Work out the finished part from the listing and answer in its coordinate system (mm). A direction names the side the tool comes from. Coordinates: 2 decimals unless noted, no trailing zeros. Loops run counter-clockwise (first coordinate to the right, second up) from the corner with the lowest first, then second, coordinate; pieces in that order, holes last. Notation, with made-up numbers: (-33.75, 33.5) -> (22.25, 33.5) arc R20 cw to (22.25, 54.5) -> close; hole circle Ø5 at (9, 21.25). An arc over 180 degrees is marked (long way). Use a Markdown table: item, result. Add a question column.
```python
from build123d import *

# Parameters (mm, degrees)
BOSS_EXTRUDE1_DEPTH = 10
SKETCH3_R           = 0.8
CUT_EXTRUDE1_DEPTH  = 10
SHELL3_START        = 0.5
SHELL3_DEPTH        = 9


# Read off the part's stored shape, not the designer's step: Shell3
with BuildPart() as part:
    # Sketch1 → Boss-Extrude1 (new body)
    with BuildSketch(Plane.XY):
        Polygon((0, 0), (17.18164136, 13.403124393), (36.182713788, 0), (31.388050652, 0), (17.18164136, 10.021027584), (3.469055949, -0.675941592), align=None)
    extrude(amount=BOSS_EXTRUDE1_DEPTH)

    # Sketch3 → Cut-Extrude1 (cut)
    with BuildSketch(Plane.XY.offset(10)):
        with Locations((3.03145353, 0.822261973)):
            Circle(SKETCH3_R)
    extrude(amount=-CUT_EXTRUDE1_DEPTH, mode=Mode.SUBTRACT)

    # Shell3 outline → Shell3 (cut)
    with BuildSketch(Plane.XY.offset(SHELL3_START)):
        with BuildLine():
            ThreePointArc((2.871909903, 1.606191709), (3.523511931, 0.19148584), (2.309922075, 1.167793967))
            Line((2.309922075, 1.167793967), (0.650444145, -0.126738299))
            Line((0.650444145, -0.126738299), (2.818611804, -0.549203293))
            Line((2.818611804, -0.549203293), (17.16665434, 10.643475851))
            Line((17.16665434, 10.643475851), (31.546653635, 0.5))
            Line((31.546653635, 0.5), (34.606450873, 0.5))
            Line((34.606450873, 0.5), (17.196628379, 12.780676126))
            Line((17.196628379, 12.780676126), (2.871909903, 1.606191709))
        make_face()
    extrude(amount=SHELL3_DEPTH, mode=Mode.SUBTRACT)


solid = part.part
```
Item 1: Find the intervals of material crossed by probe 1 along X at (y, z) = (5.75, 6.75); probe 2 along X at (y, z) = (3.5, 9.25); probe 3 along Z at (x, y) = (23.5, 8), in increasing order.
Item 2: Given pin 1 (1.5 mm diameter, centred on x = 25, y = 9, fed in from -Z); pin 2 (1 mm diameter, centred on x = 13, z = 6, fed in from -Y); pin 3 (5.5 mm diameter, centred on x = 35, z = 6.5, fed in from -Y); pin 4 (5 mm diameter, centred on y = 8, z = 1.5, fed in from -X), each flat-ended and moving along its own axis, determine where each tip first touches the part or whether it passes through.
Item 3: Section A-A (y = 4.25) is taken. Determine the outline of the cut face in (x, z).
Item 4: For faces 1 (the face through (1.49, 0.53, 4.94)), 2 (the face through (24.384, 4.94, 4.93)), 3 (the face through (21, 8, 0)), 4 (the face through (10.13, 7.27, 4.94)), 5 (the face through (26.549, 6.795, 4.93)), determine the directions among +Z, -Z, +X, -X, +Y, -Y from which every point of the face is accessible in a straight line to the end or side of a thin tool.
Item 5: Section B-B (x = 22) is taken. Determine the outline of the cut face in (y, z), then the cut area to 3 significant figures.
Item 6: Section D-D (x = 34) is taken. Determine the outline of the cut face in (y, z), then the cut area to 3 significant figures.
Item 7: For a pull along Y with two mould halves and no side action, classify faces 6 (the face through (20, 9, 0.5)), 7 (the face through (2.56, 1.47, 5.02)), 8 (the face through (21, 8, 10)), 9 (the face through (34, 0, 5)) as +Y half, -Y half, draft (parallel to the pull), parting line (faces both ways), or undercut.
Item 8: Section C-C (z = 4.75) is taken. Determine the outline of the cut face in (x, y).
Output:
| question | item | result |
|---|---|---|
| 1 | probe 1 | x = 7.37 to 8.18, 10.89 to 11.71, 23.24 to 24.1, 27.16 to 28.03 |
| 1 | probe 2 | x = 4.49 to 5.3, 8.01 to 8.82, 26.43 to 27.29, 30.35 to 31.22 |
| 1 | probe 3 | z = 0 to 0.5, 9.5 to 10 |
| 2 | pin 1 | passes through |
| 2 | pin 2 | stops at y = 6.37 |
| 2 | pin 3 | stops at y = 0 |
| 2 | pin 4 | stops at x = 7.05 |
| 3 | outline | (5.45, 0) -> (9.78, 0) -> (9.78, 10) -> (5.45, 10) -> close; (25.36, 0) -> (30.16, 0) -> (30.16, 10) -> (25.36, 10) -> close; hole (6.26, 0.5) -> (8.97, 0.5) -> (8.97, 9.5) -> (6.26, 9.5) -> close; hole (26.23, 0.5) -> (29.29, 0.5) -> (29.29, 9.5) -> (26.23, 9.5) -> close |
| 4 | face 1 | -Y |
| 4 | face 2 | +Z, -Z, -Y |
| 4 | face 3 | -Z, +X, -X, +Y, -Y |
| 4 | face 4 | none |
| 4 | face 5 | +Z, -Z, +X, +Y |
| 5 | outline | (6.62, 0) -> (10, 0) -> (10, 10) -> (6.62, 10) -> close; hole (7.23, 0.5) -> (9.39, 0.5) -> (9.39, 9.5) -> (7.23, 9.5) -> close |
| 5 | area | 14.4 mm2 |
| 6 | outline | (0, 0) -> (1.54, 0) -> (1.54, 10) -> (0, 10) -> close; hole (0.5, 0.5) -> (0.93, 0.5) -> (0.93, 9.5) -> (0.5, 9.5) -> close |
| 6 | area | 11.5 mm2 |
| 7 | face 6 | undercut |
| 7 | face 7 | undercut |
| 7 | face 8 | draft |
| 7 | face 9 | -Y half |
| 8 | outline | (0, 0) -> (0.65, -0.13) -> (2.31, 1.17) arc R0.8 cw to (2.87, 1.61) -> (17.2, 12.78) -> (34.61, 0.5) -> (31.55, 0.5) -> (17.17, 10.64) -> (2.82, -0.55) -> (3.47, -0.68) -> (17.18, 10.02) -> (31.39, 0) -> (36.18, 0) -> (17.18, 13.4) -> close |
